```python
from build123d import *

# Parameters (mm, degrees)
POCKET_DEPTH = 6.06


with BuildPart() as part:
    # Sketch → Revolve (revolve)
    with BuildSketch(Plane.YZ):
        with BuildLine():
            Line((3.999, 0), (6.5, 0))
            Line((6.5, 0), (6.5, 7.97229))
            ThreePointArc((6.5, 7.97229), (6.491884, 7.991884), (6.47229, 8))
            Line((6.47229, 8), (0, 8))
            Line((0, -30), (0, 8))
            Line((2.75, -30), (0, -30))
            Line((4, -28.75), (2.75, -30))
            Line((4, -2), (4, -28.75))
            Line((3.999, 0), (4, -2))
        make_face()
    revolve(axis=Axis((0, 0, 0), (0, 0, 1)))

    # Sketch001 → Pocket (cut)
    with BuildSketch(Plane.XY.offset(8)):
        Polygon((3.498743, 0), (1.749371, 3.03), (-1.749371, 3.03), (-3.498743, 0), (-1.749371, -3.03), (1.749371, -3.03), align=None)
    extrude(amount=-POCKET_DEPTH, mode=Mode.SUBTRACT)


solid = part.part
```
The model under review builds one solid part; all positions refer to its coordinate system, in mm. A direction names the side the tool comes from. Round coordinates to 2 decimals unless told otherwise and drop trailing zeros. Write each loop counter-clockwise with the first axis right and the second up, starting at its lowest first coordinate (ties: lowest second). Pieces come first, ordered by that corner, then holes.
(1) Insertion check: pin 1 (3 mm diameter, centred on x = -0.5, y = 1, fed in from +Z); pin 2 (5 mm diameter, centred on y = 4.5, z = -24, fed in from -X); pin 3 (3 mm diameter, centred on y = 0, z = -3, fed in from +X); pin 4 (3 mm diameter, centred on x = -0.5, z = 5, fed in from +Y). Each pin has a flat end and moves straight along its axis. Give the tip position at first contact, or say it passes through.
(2) Wall thickness on L1, parallel to Z at x = -3.75, y = 5; L2, parallel to Z at x = -2, y = 1.5; L3, parallel to X at y = 2.75, z = 2.5: over which ranges is each line inside the solid? List them lowest first.
(3) Machinability: for faces 1 (the flat face through (-3, -3, 0)), 2 (the flat face through (0, 3.03, 5)), 3 (the flat face through (3, -2, 8)), which of the approach directions +Z, -Z, +X, -X, +Y, -Y give a long, thin tool a straight path to every point of the face, cutting with its end or side? Answer none if there is none.
(4) Mouldability with a two-part tool opening along X and no side actions: class faces 4 (the flat face through (0, 0, -30)), 5 (the flat face through (2.61, -1.54, 5.01)), 6 (the conical face through (-3.372, 2.15, -1.014)) as +X half, -X half, draft (parallel to the pull), parting line (faces both ways), or undercut.
(5) We need section A-A on z = -10. Give the boundary of the cut face in (x, y), and give its area (3 significant figures).
Findings below:
1. pin 1: stops at z = 1.94
1. pin 2: stops at x = -3.46
1. pin 3: stops at x = 4
1. pin 4: stops at y = 6.5
2. L1: z = 0 to 8
2. L2: z = -30 to 1.94
2. L3: x = -5.89 to -1.91, 1.91 to 5.89
3. face 1: -Z
3. face 2: +Z
3. face 3: +Z, +X, -X, +Y, -Y
4. face 4: draft
4. face 5: undercut
4. face 6: parting line
5. outline: circle Ø8 at (0, 0)
5. area: 50.3 mm2
